Model file for the job. Use its own axes, mm. A direction names the side the tool comes from. Round coordinates to 2 decimals unless told otherwise and drop trailing zeros. Loops run counter-clockwise (first coordinate to the right, second up) from the corner with the lowest first, then second, coordinate; pieces in that order, holes last. Notation, with made-up numbers: (49, -12) -> (61, -12) arc R26 ccw to (61, 27) -> close; hole circle Ø3 at (-12.5, 59). An arc over 180 degrees is marked (long way). Use a Markdown table: item, result.
from build123d import *

# Parameters (mm, degrees)
F1_DEPTH = 1219.2
F2_W     = 76.2
F2_H     = 95.25
F3_DEPTH = 25.4
F4_R     = 7.14375
F5_DEPTH = 25.4


with BuildPart() as f1:
    # F0 (on Right) → F1 (new body)
    with BuildSketch(Plane.YZ):
        Polygon((0, 95.25), (-6.35, 95.25), (-6.35, -6.35), (69.85, -6.35), (69.85, 0), (0, 0), align=None)
    extrude(amount=F1_DEPTH)

    # F2 (on face) → F3 (cut)
    with BuildSketch(Plane.XZ.offset(6.35)):
        with Locations((38.1, 47.625)):
            Rectangle(F2_W, F2_H)
    extrude(amount=-F3_DEPTH, mode=Mode.SUBTRACT)

    # F4 (on face) → F5 (cut)
    with BuildSketch(Plane.XY):
        with Locations((32.54375, 31.75)):
            Circle(F4_R)
    extrude(amount=-F5_DEPTH, mode=Mode.SUBTRACT)


solid = f1.part
Q1. Drill centre lines: L1, parallel to X at y = 31, z = -3; L2, parallel to Z at x = 573, y = 36.5. Where is each one in solid material? Low to high. Write a range as from..to.
Results list:
| item | result |
|---|---|
| L1 | x = 0..25.44, 39.65..1219.2 |
| L2 | z = -6.35..0 |
Q2. Flat gauge pins, fed straight in: pin 1 (2 mm diameter, centred on x = 960, y = 10, fed in from +Z); pin 2 (3 mm diameter, centred on y = -2.5, z = 47.5, fed in from -X); pin 3 (10 mm diameter, centred on x = 192, z = 7, fed in from +Y). Where does each tip first touch, or does it go through?
Results list:
| item | result |
|---|---|
| pin 1 | stops at z = 0 |
| pin 2 | stops at x = 76.2 |
| pin 3 | stops at y = 0 |
Q3. Tool access for faces 1 (the face through (640, 0, 47)), 2 (the face through (737, -6.35, 45)): list every direction of +Z, -Z, +X, -X, +Y, -Y with a clear straight run to the whole face (end or side of a thin tool).
Results list:
| item | result |
|---|---|
| face 1 | +Z, +X, -X, +Y |
| face 2 | +Z, -Z, +X, -X, -Y |
Q4. Band-saw the part on B-B, the plane x = 388. Give the cut face in (y, z), plus the area to 3 significant figures.
Results list:
| item | result |
|---|---|
| outline | (-6.35, -6.35) -> (69.85, -6.35) -> (69.85, 0) -> (0, 0) -> (0, 95.25) -> (-6.35, 95.25) -> close |
| area | 1,090 mm² |
Q5. Band-saw the part on A-A, the plane z = 70.5. Give the cut face in (x, y).
Results list:
| item | result |
|---|---|
| outline | (76.2, -6.35) -> (1219.2, -6.35) -> (1219.2, 0) -> (76.2, 0) -> close |
